```python
from build123d import *

# Parameters (mm, degrees)
BOSS_EXTRUDE1_DEPTH = 50
FILLET2_R           = 10
SKETCH18_R          = 12.5
BOSS_EXTRUDE2_DEPTH = 5
SKETCH19_R          = 10.05
BOSS_EXTRUDE3_DEPTH = 30
FILLET1_R           = 10


# Read off the part's stored shape, not the designer's step: M5 Clearance Hole3
with BuildPart() as part:
    # Sketch1 → Boss-Extrude1 (new body)
    with BuildSketch(Plane(origin=(0, 0, 0), x_dir=(1, 0, 0), z_dir=(0, 1, 0))):
        Polygon((15, 15), (15, 250), (0, 250), (0, 0), (95.440306509, 0), (95.440306509, 15), align=None)
        Polygon((40.440306509, 15), (15, 99.801021696), (15, 65), (30, 15), align=None)
    extrude(amount=BOSS_EXTRUDE1_DEPTH)

    # Fillet2
    fillet2_edges = [part.edges().sort_by_distance(p)[0] for p in [
        (0, 25, 0),
    ]]
    fillet(fillet2_edges, radius=FILLET2_R)

    # M5 Clearance Hole3 outline → M5 Clearance Hole3 (revolve, cut)
    with BuildSketch(Plane(origin=(55.440306509, 40, 0), x_dir=(1, 0, 0), z_dir=(0, -1, 0))):
        Polygon((2.75, -14.975), (2.75, 0), (0, 0), (0, -15), (2.775, -15), align=None)
    revolve(axis=Axis((55.440306509, 40, 0), (0, 0, 1)), mode=Mode.SUBTRACT)

    # M5 Clearance Hole3 2 outline → M5 Clearance Hole3 2 (revolve, cut)
    with BuildSketch(Plane(origin=(85.440306509, 10, 0), x_dir=(1, 0, 0), z_dir=(0, -1, 0))):
        Polygon((2.75, -14.975), (2.75, 0), (0, 0), (0, -15), (2.775, -15), align=None)
    revolve(axis=Axis((85.440306509, 10, 0), (0, 0, 1)), mode=Mode.SUBTRACT)

    # M5 Clearance Hole3 3 outline → M5 Clearance Hole3 3 (revolve, cut)
    with BuildSketch(Plane(origin=(55.440306509, 10, 0), x_dir=(1, 0, 0), z_dir=(0, -1, 0))):
        Polygon((2.75, -14.975), (2.75, 0), (0, 0), (0, -15), (2.775, -15), align=None)
    revolve(axis=Axis((55.440306509, 10, 0), (0, 0, 1)), mode=Mode.SUBTRACT)

    # M5 Clearance Hole3 4 outline → M5 Clearance Hole3 4 (revolve, cut)
    with BuildSketch(Plane(origin=(85.440306509, 40, 0), x_dir=(1, 0, 0), z_dir=(0, -1, 0))):
        Polygon((2.75, -14.975), (2.75, 0), (0, 0), (0, -15), (2.775, -15), align=None)
    revolve(axis=Axis((85.440306509, 40, 0), (0, 0, 1)), mode=Mode.SUBTRACT)

    # Sketch18 → Boss-Extrude2 (add)
    with BuildSketch(Plane.ZY):
        with Locations(Location((-210, 25, 0), (0, 0, 180))):
            Circle(SKETCH18_R)
    extrude(amount=BOSS_EXTRUDE2_DEPTH)

    # Sketch19 → Boss-Extrude3 (add)
    with BuildSketch(Plane.ZY.offset(5)):
        with Locations((-210, 25)):
            Circle(SKETCH19_R)
    extrude(amount=BOSS_EXTRUDE3_DEPTH)

    # Fillet1
    fillet1_edges = [part.edges().sort_by_distance(p)[0] for p in [
        (95.440306509, 0, -7.5),
        (7.5, 0, -250),
        (7.5, 50, -250),
        (95.440306509, 50, -7.5),
    ]]
    fillet(fillet1_edges, radius=FILLET1_R)


solid = part.part
```
Here's how the part is built. I have some questions about the finished solid (model axes, mm). A direction names the side the tool comes from. Give positions to 0.01 mm unless a question says otherwise; leave off trailing zeros. Loops run counter-clockwise (first coordinate to the right, second up) from the corner with the lowest first, then second, coordinate; pieces in that order, holes last. Notation, with made-up numbers: (47.25, 14.25) -> (98.25, 14.25) arc R23 ccw to (98.25, 26.25) -> close; hole circle Ø3 at (-5, 35.5). An arc over 180 degrees is marked (long way). Use one line per item in the form item = value. Start each with the question number.
1) For P1, Ø5, axis at x = -15.5, z = -199.5, coming from the -Y side; P2, Ø6.5, axis at x = 85.44, y = 40, coming from the -Z side; P3, Ø15, axis at y = 12.5, z = -206, coming from the +X side; P4, Ø4.5, axis at x = 55.44, y = 10, coming from the +Z side, each with a flat end and sliding along its axis, tell me the tip position at first contact or that it passes through.
2) Imagine slicing it at D-D (z = -210). Please give me the cut outline in (x, y), then the cut area to 3 significant figures.
3) Imagine slicing it at A-A (y = 25). Please give me the cut outline in (x, z).
4) Imagine slicing it at B-B (z = -23). Please give me the cut outline in (x, y), then the cut area to 3 significant figures.
5) Which directions (+Z, -Z, +X, -X, +Y, -Y) give clear straight access to the entire face, cutting with the end or side of a thin tool? Please do faces 1 (the face through (52.693, 10.121, -7.383)), 2 (the face through (-19.79, 18.885, -217.975)).
6) Thinking about a two-plate mould opening in Y: for faces 3 (the face through (-2.465, 21.245, -221.923)), 4 (the face through (0, 25, -132)), 5 (the face through (82.693, 10.121, -7.383)), which applies, +Y half, -Y half, draft (parallel to the pull), parting line (faces both ways), or undercut?
7) Imagine slicing it at C-C (x = -22). Please give me the cut outline in (y, z).
8) Please list where these lines run through material, in increasing order: line 1 along X through (y, z) = (7.5, -11.5); line 2 along X through (y, z) = (42.5, -112); line 3 along Z through (x, y) = (81, 43).
Check values:
q1.P1 = 18.92
q1.P2 = -15
q1.P3 = 15
q1.P4 = through
q2.outline = (-35, 14.95) -> (-5, 14.95) -> (-5, 12.5) -> (0, 12.5) -> (0, 0) -> (15, 0) -> (15, 50) -> (0, 50) -> (0, 37.5) -> (-5, 37.5) -> (-5, 35.05) -> (-35, 35.05) -> close
q2.area = 1,480 mm^2
q3.outline = (-35, -220.05) -> (-5, -220.05) -> (-5, -222.5) -> (0, -222.5) -> (0, -250) -> (15, -250) -> (15, -99.8) -> (40.44, -15) -> (95.44, -15) -> (95.44, 0) -> (10, 0) arc R10 ccw to (0, -10) -> (0, -197.5) -> (-5, -197.5) -> (-5, -199.95) -> (-35, -199.95) -> close; hole (15, -65) -> (30, -15) -> (15, -15) -> close
q4.outline = (0, 0) -> (15, 0) -> (15, 50) -> (0, 50) -> close; (27.6, 0) -> (38.04, 0) -> (38.04, 50) -> (27.6, 50) -> close
q4.area = 1,270 mm^2
q5.face_1 = +Z, -Z
q5.face_2 = -X
q6.face_3 = parting line
q6.face_4 = draft
q6.face_5 = undercut
q7.outline = circle Ø20.1 at (25, -210)
q8.line_1 = 0 to 54.29, 56.59 to 84.29, 86.59 to 95.12
q8.line_2 = 0 to 15
q8.line_3 = -15 to 0
